Part model, mm, in its own coordinate system. Face numbers are marked on the shaded views. A direction names the side the tool comes from. Give positions to 0.01 mm unless a question says otherwise; leave off trailing zeros. Loops run counter-clockwise (first coordinate to the right, second up) from the corner with the lowest first, then second, coordinate; pieces in that order, holes last. Notation, with made-up numbers: M 69.25,85.5 L 99.25,85.5 A24 cw 99.25,105.5 Z; hole C -1.75,-6 d9. An arc over 180 degrees is marked long. Answer in a Markdown table with one row per item.
from build123d import *

# Parameters (mm, degrees)
F0_W     = 150.792748
F0_H     = 102.713902
F1_DEPTH = 76.2
F3_DEPTH = 50.8
F5_DEPTH = 50.8
F7_DEPTH = 25.4


with BuildPart() as f1:
    # F0 (on Front) → F1 (new body)
    with BuildSketch(Plane.XZ):
        with Locations((-0.485644, 4.735036)):
            Rectangle(F0_W, F0_H)
    extrude(amount=F1_DEPTH)

    # F2 (on face) → F3 (cut)
    with BuildSketch(Plane.YZ.offset(74.91073)):
        Polygon((-76.2, 56.091987), (-76.2, -46.621915), (0, 56.091987), align=None)
    extrude(amount=-F3_DEPTH, mode=Mode.SUBTRACT)

    # F4 (on face) → F5 (cut)
    with BuildSketch(Plane(origin=(-75.882018, 0, 0), x_dir=(0, -1, 0), z_dir=(-1, 0, 0))):
        Polygon((76.2, 56.091987), (0, 56.091987), (76.2, -46.621915), align=None)
    extrude(amount=-F5_DEPTH, mode=Mode.SUBTRACT)

    # F6 (on face) → F7 (join)
    with BuildSketch(Plane(origin=(0, 0, 0), x_dir=(-1, 0, 0), z_dir=(0, 1, 0))):
        Polygon((-24.11073, 56.091987), (-74.91073, 56.091987), (-74.91073, -46.621915), (75.882018, -46.621915), (75.882018, 56.091987), (25.082018, 56.091987), align=None)
    extrude(amount=F7_DEPTH)


solid = f1.part
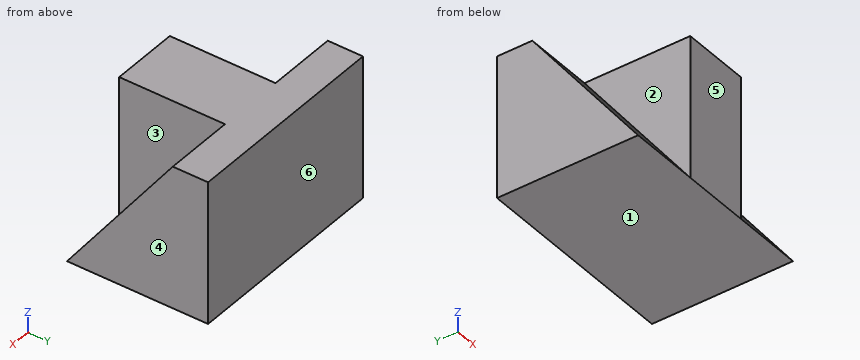
(1) Pin check, flat tips, straight feed: pin 1 Ø2 at (x, z) = (48, -31) entering from -Y; pin 2 Ø8 at (x, z) = (-41, 20.5) entering from -Y. Stop position of each tip, or through.
Recorded:
| item | result |
|---|---|
| pin 1 | stops at y = -65.35 |
| pin 2 | stops at y = -29.37 |
(2) Which spindle directions (+Z, -Z, +X, -X, +Y, -Y) get a long thin tool onto all of the face, cutting with end or side? Do the marked faces 1, 2 and 3. Say none if no direction does.
Recorded:
| item | result |
|---|---|
| face 1 | -Z, +X, -X, +Y, -Y |
| face 2 | +Z, -X, -Y |
| face 3 | +Z, +X, -Y |
(3) Pull direction Y, two halves, no side cores. Call the marked faces 4, 5 and 6: +Y half, -Y half, draft (parallel to the pull), parting line (faces both ways), or undercut.
Recorded:
| item | result |
|---|---|
| face 4 | draft |
| face 5 | -Y half |
| face 6 | +Y half |
(4) Saw through at C-C (x = 52). Write the cut outline in (y, z).
Recorded:
| item | result |
|---|---|
| outline | M -76.2,-46.62 L 25.4,-46.62 L 25.4,56.09 L 0,56.09 Z |
(5) Saw through at A-A (z = 26.5). Write the cut outline in (x, y).
Recorded:
| item | result |
|---|---|
| outline | M -75.88,-21.95 L -25.08,-21.95 L -25.08,-76.2 L 24.11,-76.2 L 24.11,-21.95 L 74.91,-21.95 L 74.91,25.4 L -75.88,25.4 Z |
(6) Saw through at B-B (y = -12). Write the cut outline in (x, z).
Recorded:
| item | result |
|---|---|
| outline | M -75.88,-46.62 L 74.91,-46.62 L 74.91,39.92 L 24.11,39.92 L 24.11,56.09 L -25.08,56.09 L -25.08,39.92 L -75.88,39.92 Z |
(7) Drill centre lines: line 1 along X through (y, z) = (-33, 38); line 2 along Y through (x, z) = (35, 10); line 3 along Z through (x, y) = (54, -23.5). Where is each one in solid material? Low to high.
Recorded:
| item | result |
|---|---|
| line 1 | x = -25.08 to 24.11 |
| line 2 | y = -34.19 to 25.4 |
| line 3 | z = -46.62 to 24.42 |
